from build123d import *

# Parameters (mm, degrees)
CYLINDER081_R          = 4
CYLINDER081_DEPTH      = 10
BOX058_W               = 4
BOX058_H               = 4
BOX058_DEPTH           = 10
CUT030_PLACEMENT_ANGLE = 180
CYLINDER077_R          = 3
CYLINDER077_DEPTH      = 10
BOX054_W               = 3
BOX054_H               = 3
BOX054_DEPTH           = 10
CYLINDER078_R          = 3
CYLINDER078_DEPTH      = 10
BOX055_W               = 3
BOX055_H               = 3
BOX055_DEPTH           = 10
CUT027_PLACEMENT_ANGLE = 270
CYLINDER080_R          = 4
CYLINDER080_DEPTH      = 10
BOX057_W               = 4
BOX057_H               = 4
BOX057_DEPTH           = 10
CUT029_PLACEMENT_ANGLE = 90
BOX053_W               = 73
BOX053_H               = 58
BOX053_DEPTH           = 10
CYLINDER074_R          = 12
CYLINDER074_DEPTH      = 10
BOX050_W               = 12
BOX050_H               = 12
BOX050_DEPTH           = 4
CUT022_PLACEMENT_ANGLE = 90
CYLINDER075_R          = 12
CYLINDER075_DEPTH      = 10
BOX051_W               = 12
BOX051_H               = 12
BOX051_DEPTH           = 4
CUT023_PLACEMENT_ANGLE = 180
CYLINDER076_R          = 12
CYLINDER076_DEPTH      = 10
BOX052_W               = 12
BOX052_H               = 12
BOX052_DEPTH           = 4
CUT024_PLACEMENT_ANGLE = 90
CYLINDER073_R          = 12
CYLINDER073_DEPTH      = 10
BOX049_W               = 12
BOX049_H               = 12
BOX049_DEPTH           = 4
BOX048_W               = 140
BOX048_H               = 113
BOX048_DEPTH           = 4


with BuildPart() as cylinder083:
    # Cylinder081 → Cylinder081 (new body)
    with BuildSketch(Plane(origin=(36.5, 67, 26), x_dir=(1, 0, 0), z_dir=(0, 0, 1))):
        Circle(CYLINDER081_R)
    extrude(amount=CYLINDER081_DEPTH)


with BuildPart() as obj1:
    # Box058 → Box058 (new body)
    with BuildSketch(Plane(origin=(32.5, 67, 26), x_dir=(1, 0, 0), z_dir=(0, 0, 1))):
        with Locations((2, 2)):
            Rectangle(BOX058_W, BOX058_H)
    extrude(amount=BOX058_DEPTH)

    # Cut030: cut Cylinder083
    add(cylinder083.part, mode=Mode.SUBTRACT)


with BuildPart() as obj1_1:
    # Cut030 placement: moved
    add(obj1.part.moved(Location((139, 83, 0))).rotate(Axis((139, 83, 0), (0, 0, 1)), CUT030_PLACEMENT_ANGLE))


with BuildPart() as cylinder079:
    # Cylinder077 → Cylinder077 (new body)
    with BuildSketch(Plane(origin=(36.5, 67, 26), x_dir=(1, 0, 0), z_dir=(0, 0, 1))):
        Circle(CYLINDER077_R)
    extrude(amount=CYLINDER077_DEPTH)


with BuildPart() as obj2:
    # Box054 → Box054 (new body)
    with BuildSketch(Plane(origin=(33.5, 67, 26), x_dir=(1, 0, 0), z_dir=(0, 0, 1))):
        with Locations((1.5, 1.5)):
            Rectangle(BOX054_W, BOX054_H)
    extrude(amount=BOX054_DEPTH)

    # Cut026: cut Cylinder079
    add(cylinder079.part, mode=Mode.SUBTRACT)


with BuildPart() as cylinder080:
    # Cylinder078 → Cylinder078 (new body)
    with BuildSketch(Plane(origin=(36.5, 67, 26), x_dir=(1, 0, 0), z_dir=(0, 0, 1))):
        Circle(CYLINDER078_R)
    extrude(amount=CYLINDER078_DEPTH)


with BuildPart() as obj3:
    # Box055 → Box055 (new body)
    with BuildSketch(Plane(origin=(33.5, 67, 26), x_dir=(1, 0, 0), z_dir=(0, 0, 1))):
        with Locations((1.5, 1.5)):
            Rectangle(BOX055_W, BOX055_H)
    extrude(amount=BOX055_DEPTH)

    # Cut027: cut Cylinder080
    add(cylinder080.part, mode=Mode.SUBTRACT)


with BuildPart() as obj3_1:
    # Cut027 placement: moved
    add(obj3.part.moved(Location((36.5, 103.5, 0))).rotate(Axis((36.5, 103.5, 0), (0, 0, 1)), CUT027_PLACEMENT_ANGLE))


with BuildPart() as cylinder082:
    # Cylinder080 → Cylinder080 (new body)
    with BuildSketch(Plane(origin=(36.5, 67, 26), x_dir=(1, 0, 0), z_dir=(0, 0, 1))):
        Circle(CYLINDER080_R)
    extrude(amount=CYLINDER080_DEPTH)


with BuildPart() as displaycuts:
    # Box057 → Box057 (new body)
    with BuildSketch(Plane(origin=(32.5, 67, 26), x_dir=(1, 0, 0), z_dir=(0, 0, 1))):
        with Locations((2, 2)):
            Rectangle(BOX057_W, BOX057_H)
    extrude(amount=BOX057_DEPTH)

    # Cut029: cut Cylinder082
    add(cylinder082.part, mode=Mode.SUBTRACT)


with BuildPart() as displaycuts_1:
    # Cut029 placement: moved
    add(displaycuts.part.moved(Location((104.5, -20.5, 0))).rotate(Axis((104.5, -20.5, 0), (0, 0, 1)), CUT029_PLACEMENT_ANGLE))

    # Fusion041: union obj1, obj2, obj3
    add(obj1_1.part)
    add(obj2.part)
    add(obj3_1.part)


with BuildPart() as topcut:
    # Box053 → Box053 (new body)
    with BuildSketch(Plane(origin=(33.5, 12, 26), x_dir=(1, 0, 0), z_dir=(0, 0, 1))):
        with Locations((36.5, 29)):
            Rectangle(BOX053_W, BOX053_H)
    extrude(amount=BOX053_DEPTH)

    # Cut031: cut displayCuts
    add(displaycuts_1.part, mode=Mode.SUBTRACT)


with BuildPart() as cylinder076:
    # Cylinder074 → Cylinder074 (new body)
    with BuildSketch(Plane(origin=(12, 12, 0), x_dir=(1, 0, 0), z_dir=(0, 0, 1))):
        Circle(CYLINDER074_R)
    extrude(amount=CYLINDER074_DEPTH)


with BuildPart() as cutout006:
    # Box050 → Box050 (new body)
    with BuildSketch(Plane.XY):
        with Locations((6, 6)):
            Rectangle(BOX050_W, BOX050_H)
    extrude(amount=BOX050_DEPTH)

    # Cut022: cut Cylinder076
    add(cylinder076.part, mode=Mode.SUBTRACT)


with BuildPart() as cutout006_1:
    # Cut022 placement: moved
    add(cutout006.part.moved(Location((140, 0, 0))).rotate(Axis((140, 0, 0), (0, 0, 1)), CUT022_PLACEMENT_ANGLE))


with BuildPart() as cylinder077:
    # Cylinder075 → Cylinder075 (new body)
    with BuildSketch(Plane(origin=(12, 12, 0), x_dir=(1, 0, 0), z_dir=(0, 0, 1))):
        Circle(CYLINDER075_R)
    extrude(amount=CYLINDER075_DEPTH)


with BuildPart() as cutout007:
    # Box051 → Box051 (new body)
    with BuildSketch(Plane.XY):
        with Locations((6, 6)):
            Rectangle(BOX051_W, BOX051_H)
    extrude(amount=BOX051_DEPTH)

    # Cut023: cut Cylinder077
    add(cylinder077.part, mode=Mode.SUBTRACT)


with BuildPart() as cutout007_1:
    # Cut023 placement: moved
    add(cutout007.part.moved(Location((140, 113, 0))).rotate(Axis((140, 113, 0), (0, 0, 1)), CUT023_PLACEMENT_ANGLE))


with BuildPart() as cylinder078:
    # Cylinder076 → Cylinder076 (new body)
    with BuildSketch(Plane(origin=(12, 12, 0), x_dir=(1, 0, 0), z_dir=(0, 0, 1))):
        Circle(CYLINDER076_R)
    extrude(amount=CYLINDER076_DEPTH)


with BuildPart() as cutout008:
    # Box052 → Box052 (new body)
    with BuildSketch(Plane.XY):
        with Locations((6, 6)):
            Rectangle(BOX052_W, BOX052_H)
    extrude(amount=BOX052_DEPTH)

    # Cut024: cut Cylinder078
    add(cylinder078.part, mode=Mode.SUBTRACT)


with BuildPart() as cutout008_1:
    # Cut024 placement: moved
    add(cutout008.part.moved(Location((0, 113, 0))).rotate(Axis((0, 113, 0), (0, 0, -1)), CUT024_PLACEMENT_ANGLE))


with BuildPart() as cylinder075:
    # Cylinder073 → Cylinder073 (new body)
    with BuildSketch(Plane(origin=(12, 12, 0), x_dir=(1, 0, 0), z_dir=(0, 0, 1))):
        Circle(CYLINDER073_R)
    extrude(amount=CYLINDER073_DEPTH)


with BuildPart() as cutout009:
    # Box049 → Box049 (new body)
    with BuildSketch(Plane.XY):
        with Locations((6, 6)):
            Rectangle(BOX049_W, BOX049_H)
    extrude(amount=BOX049_DEPTH)

    # Cut021: cut Cylinder075
    add(cylinder075.part, mode=Mode.SUBTRACT)

    # Fusion040: union cutOut006, cutOut007, cutOut008
    add(cutout006_1.part)
    add(cutout007_1.part)
    add(cutout008_1.part)


with BuildPart() as top002:
    # Box048 → Box048 (new body)
    with BuildSketch(Plane.XY):
        with Locations((70, 56.5)):
            Rectangle(BOX048_W, BOX048_H)
    extrude(amount=BOX048_DEPTH)

    # Cut025: cut cutOut009
    add(cutout009.part, mode=Mode.SUBTRACT)


with BuildPart() as top002_1:
    # Cut025 placement: moved
    add(top002.part.moved(Location((0, 0, 26))))

    # Cut032: cut topCut
    add(topcut.part, mode=Mode.SUBTRACT)


solid = top002_1.part
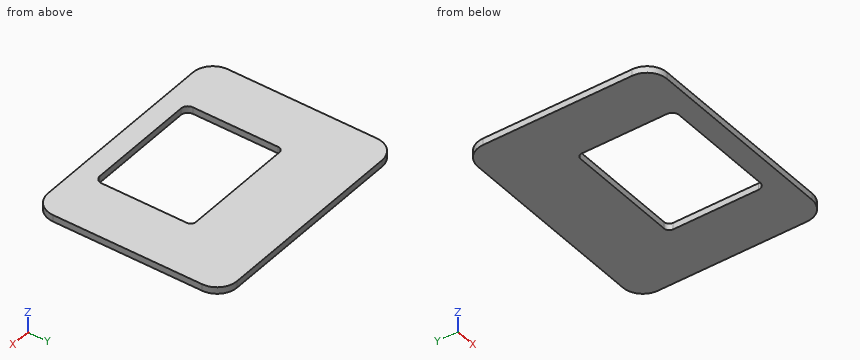
Read the model definition and answer for the solid it produces. Units are mm, in the model's axes. Round coordinates to 2 decimals unless told otherwise and drop trailing zeros. Order: outer loops, then holes, each group sorted by start corner. A loop starts at its lowest first (then second) coordinate and runs counter-clockwise, first axis right, second up. Notation, with made-up numbers: (19.25, -39.75) - (51.25, -39.75) arc R14 cw to (51.25, -14.75) - close; hole circle Ø8 at (72.25, 65). An arc over 180 degrees is marked (long way). Use one line per item in the form item = value. Start each with the question number.
(1) Find the intervals of material crossed by line 1 along Y through (x, z) = (49.5, 28.25); line 2 along X through (y, z) = (20, 27.9); line 3 along Y through (x, z) = (10.5, 27.95), in increasing order. Write a range as from..to.
(2) The part is cut by section A-A (z = 27.5). Give the vertices of the cut face in (x, y).
(3) The part is cut by section B-B (y = 54). Give the vertices of the cut face in (x, z), then the cut area to 3 significant figures.
(4) The part is cut by section C-C (x = 41.5). Give the vertices of the cut face in (y, z), then the cut area to 3 significant figures.
Checked values:
q1.line_1 = 0..12, 70..113
q1.line_2 = 0..33.5, 106.5..140
q1.line_3 = 0.09..112.91
q2.outline = (0, 12) arc R12 ccw to (12, 0) - (128, 0) arc R12 ccw to (140, 12) - (140, 101) arc R12 ccw to (128, 113) - (12, 113) arc R12 ccw to (0, 101) - close; hole (33.5, 16) arc R4 ccw to (37.5, 12) - (102.5, 12) arc R4 ccw to (106.5, 16) - (106.5, 67) arc R3 ccw to (103.5, 70) - (36.5, 70) arc R3 ccw to (33.5, 67) - close
q3.outline = (0, 26) - (33.5, 26) - (33.5, 30) - (0, 30) - close; (106.5, 26) - (140, 26) - (140, 30) - (106.5, 30) - close
q3.area = 268 mm^2
q4.outline = (0, 26) - (12, 26) - (12, 30) - (0, 30) - close; (70, 26) - (113, 26) - (113, 30) - (70, 30) - close
q4.area = 220 mm^2
